For this review, take the finished solid that the model builds, in its own axes (mm). Face numbers are marked on the shaded views. A direction names the side the tool comes from. Round coordinates to 2 decimals unless told otherwise and drop trailing zeros. Order: outer loops, then holes, each group sorted by start corner. A loop starts at its lowest first (then second) coordinate and runs counter-clockwise, first axis right, second up. Notation, with made-up numbers: M 41.25,37 L 78.25,37 A21 ccw 78.25,42 Z; hole C 88,89 d9. An arc over 180 degrees is marked long. Put each result on its own line as item: value.
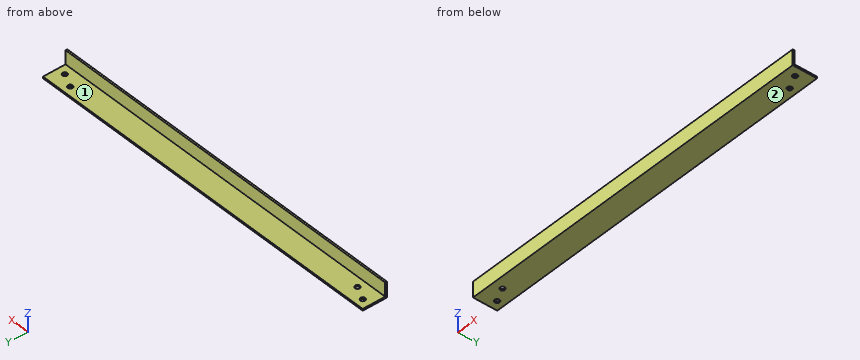
from build123d import *

# Parameters (mm, degrees)
SKETCH_1_W          = 1675
SKETCH_1_H          = 110
EXTRUDE_1_DEPTH     = 8
SKETCH_2_W          = 1675
SKETCH_2_H          = 8
EXTRUDE_2_DEPTH     = 62
SKETCH_3_R          = 11
CUT_EXTRUDE_1_DEPTH = 1681.066962951


with BuildPart() as part:
    # 草图1 → 拉伸1 (new body)
    with BuildSketch(Plane.XY):
        with Locations((837.5, 55)):
            Rectangle(SKETCH_1_W, SKETCH_1_H)
    extrude(amount=EXTRUDE_1_DEPTH)

    # 草图2 → 拉伸2 (add)
    with BuildSketch(Plane.XY.offset(8)):
        with Locations((837.5, 4)):
            Rectangle(SKETCH_2_W, SKETCH_2_H)
    extrude(amount=EXTRUDE_2_DEPTH)

    # 草图3 → 切除-拉伸1 (cut, through all)
    with BuildSketch(Plane(origin=(0, 0, 0), x_dir=(-1, 0, 0), z_dir=(0, 0, -1))):
        with Locations((-1635.574764315, 45)):
            Circle(SKETCH_3_R)
        with Locations((-1572.407333755, 75.164146207)):
            Circle(SKETCH_3_R)
        with Locations((-102.592666245, 45)):
            Circle(SKETCH_3_R)
        with Locations((-39.425235685, 75.164146207)):
            Circle(SKETCH_3_R)
    extrude(amount=-CUT_EXTRUDE_1_DEPTH, mode=Mode.SUBTRACT)


solid = part.part
(1) Add section B-B on z = 58.5. Give the boundary of the cut face in (x, y), then the cut area to 3 significant figures.
A:
outline: M 0,0 L 1675,0 L 1675,8 L 0,8 Z
area: 13,400 mm2
(2) For the marked faces 1 and 2, list the 3-axis set-ups (+Z, -Z, +X, -X, +Y, -Y) from which the entire face can be reached by the end or side of a thin tool; tool diameter is ignored.
A:
face 1: +Z, +X, -X, +Y
face 2: -Z, +X, -X, +Y, -Y
(3) To check wall thickness, follow L1, parallel to X at y = 78.5, z = 5; L2, parallel to Y at x = 1398, z = 27. State the ranges of each line that lie inside material, in increasing order.
A:
L1: x = 0 to 28.94, 49.91 to 1561.93, 1582.89 to 1675
L2: y = 0 to 8
(4) Add section A-A on x = 1368. Give the boundary of the cut face in (y, z).
A:
outline: M 0,0 L 110,0 L 110,8 L 8,8 L 8,70 L 0,70 Z
(5) Insertion check: pin 1 Ø4 at (x, y) = (589.5, 79.5) entering from +Z. The pin has a flat end and moves straight along its axis. Give the tip position at first contact, or say it passes through.
A:
pin 1: stops at z = 8
